from build123d import *

# Parameters (mm, degrees)
SKETCH_1_W          = 70
SKETCH_1_H          = 100
EXTRUDE_1_DEPTH     = 3
SKETCH_2_R          = 1.575
CUT_EXTRUDE_1_DEPTH = 123.102416029
CUT_EXTRUDE_2_DEPTH = 123.102416029
FILLET_2_R          = 3


with BuildPart() as part:
    # 草图1 → 凸台-拉伸1 (new body)
    with BuildSketch(Plane.XY):
        with Locations((35, -50)):
            Rectangle(SKETCH_1_W, SKETCH_1_H)
    extrude(amount=EXTRUDE_1_DEPTH)

    # 草图2 → 切除-拉伸1 (cut, through all)
    with BuildSketch(Plane.XY.offset(3)):
        with Locations((5, -5)):
            Circle(SKETCH_2_R)
        with Locations(Location((15, -5, 0), (0, 0, 180))):
            Circle(SKETCH_2_R)
        with Locations((15, -15)):
            Circle(SKETCH_2_R)
        with Locations(Location((5, -15, 0), (0, 0, 180))):
            Circle(SKETCH_2_R)
        with Locations((65, -15)):
            Circle(SKETCH_2_R)
        with Locations(Location((55, -15, 0), (0, 0, 180))):
            Circle(SKETCH_2_R)
        with Locations((55, -5)):
            Circle(SKETCH_2_R)
        with Locations(Location((65, -5, 0), (0, 0, 180))):
            Circle(SKETCH_2_R)
        with Locations((10, -85)):
            Circle(SKETCH_2_R)
        with Locations((35, -85)):
            Circle(SKETCH_2_R)
        with Locations(Location((60, -85, 0), (0, 0, 180))):
            Circle(SKETCH_2_R)
        with Locations((60, -75)):
            Circle(SKETCH_2_R)
        with Locations(Location((35, -75, 0), (0, 0, 180))):
            Circle(SKETCH_2_R)
        with Locations(Location((10, -75, 0), (0, 0, 180))):
            Circle(SKETCH_2_R)
        with Locations((10, -95)):
            Circle(SKETCH_2_R)
        with Locations((35, -95)):
            Circle(SKETCH_2_R)
        with Locations(Location((60, -95, 0), (0, 0, 180))):
            Circle(SKETCH_2_R)
    extrude(amount=-CUT_EXTRUDE_1_DEPTH, mode=Mode.SUBTRACT)

    # 草图3 → 切除-拉伸2 (cut, through all)
    with BuildSketch(Plane(origin=(0, 0, 0), x_dir=(-1, 0, 0), z_dir=(0, 0, -1))):
        Polygon((-65, -30), (-65, -65), (-48, -65), align=None)
        Polygon((-57, -30), (-40, -65), (-40, -30), align=None)
        Polygon((-30, -30), (-13, -30), (-30, -65), align=None)
        Polygon((-22, -65), (-5, -30), (-5, -65), align=None)
        Polygon((-35, -6), (-50, -21), (-20, -21), align=None)
    extrude(amount=-CUT_EXTRUDE_2_DEPTH, mode=Mode.SUBTRACT)

    # 圆角2
    fillet_2_edges = [part.edges().sort_by_distance(p)[0] for p in [
        (57, -30, 1.5),
        (40, -30, 1.5),
        (40, -65, 1.5),
        (30, -65, 1.5),
        (30, -30, 1.5),
        (13, -30, 1.5),
        (5, -65, 1.5),
        (22, -65, 1.5),
        (5, -30, 1.5),
        (35, -6, 1.5),
        (20, -21, 1.5),
        (50, -21, 1.5),
        (65, -30, 1.5),
        (48, -65, 1.5),
        (65, -65, 1.5),
    ]]
    fillet(fillet_2_edges, radius=FILLET_2_R)


solid = part.part
The listing builds one solid part. Answer for the finished solid, in the listing's coordinates (mm). Give positions to 0.01 mm unless a question says otherwise; leave off trailing zeros.
1) Section A-A (z = 2) is taken. Count the separate pieces of the cut face and the enclosed holes in it, and give its area (3 significant figures).
2) Find the intervals of material crossed by L1, parallel to X at y = -95, z = 2.35 (3 decimals); L2, parallel to Y at x = 36, z = 2.15; L3, parallel to Y at x = 28, z = 1.7, in increasing order.
3) For a pull along X with two mould halves and no side action, classify faces 1 (the face through (35, 0, 1)), 2 (the face through (27.617, -54.893, 1.521)) as pulls with the +X half, pulls with the -X half, needs draft (parallel to the pull), parting line crosses it, or undercut.
Response:
1. separate pieces: 1
1. enclosed holes: 22
1. area: 5,610 mm2
2. L1: x = 0 to 8.425, 11.575 to 33.425, 36.575 to 58.425, 61.575 to 70
2. L2: y = -100 to -96.22, -93.78 to -86.22, -83.78 to -76.22, -73.78 to -21, -7.41 to 0
2. L3: y = -100 to -54.79, -30.17 to -21, -13 to 0
3. face 1: needs draft
3. face 2: undercut
